Can you work these out from the model? Positions are in its coordinate system, mm. A direction names the side the tool comes from. Round coordinates to 2 decimals unless told otherwise and drop trailing zeros. Order: outer loops, then holes, each group sorted by start corner. A loop starts at its lowest first (then second) coordinate and runs counter-clockwise, first axis right, second up.
Q1. If we section it at C-C (z = 46.5): Please give me the cut outline in (x, y).
Q2. If we section it at A-A (y = 0): Please give me the cut outline in (x, z) (3 decimals), plus the area to 3 significant figures.
Q3. If we section it at B-B (x = 0): Please give me the cut outline in (y, z) (3 decimals).
Q4. Will these pins go through, and if not, where does the flat tip stop? P1, Ø16.5, axis at y = -16.5, z = 48.5, coming from the +X side; P2, Ø11.5, axis at x = -45.5, y = -11.5, coming from the +Z side; P3, Ø21.5, axis at x = 22, y = -9.5, coming from the +Z side.
Q5. We'd pull the mould along Y, two halves only. Please class faces 1 (the face through (25, 24.855, 58)), 2 (the face through (15.002, -3, 51)): pulls with the +Y half, pulls with the -Y half, needs draft (parallel to the pull), parting line crosses it, or undercut.
Q6. If we section it at D-D (z = 4): Please give me the cut outline in (x, y) (3 decimals), plus the area to 3 significant figures.
Q7. For faces 3 (the face through (-47.564, -1, 13)), 4 (the face through (58, 13.025, 13)), 5 (the face through (45, -1, 25.4)), 6 (the face through (-35.702, -2, 40)), 7 (the face through (-17.032, -40, 58)), which set-ups out of +Z, -Z, +X, -X, +Y, -Y let a thin tool reach every point of the face, with its end or its side?
Q8. If I drill on line 1 (Y direction, x = 0, z = 17) (3 decimals); line 2 (X direction, y = -41, z = 56.5); line 3 (X direction, y = 16.5, z = 49.5), over which ranges is the centre line in solid material (lowest first)?
from build123d import *

# Parameters (mm, degrees)
F0_W      = 144.9018344283
F0_H      = 100.0124998391
F1_DEPTH  = 25.4
F2_W      = 23.9564813673
F2_H      = 30.4689249024
F3_DEPTH  = 25.4
F4_W      = 27.2127054632
F4_H      = 32.7947968617
F5_DEPTH  = 25.4
F6_W      = 70.706512779
F6_H      = 100.0124998391
F7_DEPTH  = 17.78
F9_W      = 19.5373268798
F9_H      = 99.2384850979
F8_W      = 19.0721508116
F8_H      = 100.0124998391
F10_DEPTH = 10.16
F12_W     = 19.5373268798
F12_H     = 22.7496176958
F11_W     = 19.0721508116
F11_H     = 23.2910439372
F15_DEPTH = 10.16
F13_W     = 18.3743890375
F13_H     = 23.6915722489
F14_W     = 19.367502071
F14_H     = 23.0261366814
F16_DEPTH = 10.16
F19_D     = 21.59


with BuildPart() as f1:
    # F0 (on Top) → F1 (new body)
    with BuildSketch(Plane.XY):
        with Locations((-2.325873822, -1.6281101853)):
            Rectangle(F0_W, F0_H)
    extrude(amount=F1_DEPTH)

    # F2 (on face) → F3 (cut)
    with BuildSketch(Plane.XY.offset(25.4)):
        with Locations((58.1468027085, -2.2095781751)):
            Rectangle(F2_W, F2_H)
    extrude(amount=-F3_DEPTH, mode=Mode.SUBTRACT)

    # F4 (on face) → F5 (cut)
    with BuildSketch(Plane.XY.offset(25.4)):
        with Locations((-61.1704383045, -1.0466421954)):
            Rectangle(F4_W, F4_H)
    extrude(amount=-F5_DEPTH, mode=Mode.SUBTRACT)

    # F6 (on face) → F7 (join)
    with BuildSketch(Plane.XY.offset(25.4)):
        with Locations((-0.3488790244, -1.6281101853)):
            Rectangle(F6_W, F6_H)
    extrude(amount=F7_DEPTH)

    # F9 (on face) + F8 (on face) → F10 (join)
    with BuildSketch(Plane.XY.offset(43.18)):
        with Locations((24.7705369256, -2.0151175559)):
            Rectangle(F9_W, F9_H)
    with BuildSketch(Plane.XY.offset(43.18)):
        with Locations((-26.1660600081, -1.6281101853)):
            Rectangle(F8_W, F8_H)
    extrude(amount=F10_DEPTH)

    # F12 (on face) + F11 (on face) → F15 (join)
    with BuildSketch(Plane.XY.offset(53.34)):
        with Locations((24.7705369256, 36.2293161452)):
            Rectangle(F12_W, F12_H)
    with BuildSketch(Plane.XY.offset(53.34)):
        with Locations((-26.1660600081, 36.7326177657)):
            Rectangle(F11_W, F11_H)
    extrude(amount=F15_DEPTH)

    # F13 (on face) + F14 (on face) → F16 (join)
    with BuildSketch(Plane.XY.offset(53.34)):
        with Locations((-26.2195924297, -39.7885739803)):
            Rectangle(F13_W, F13_H)
    with BuildSketch(Plane.XY.offset(53.34)):
        with Locations((24.6856245212, -39.9210313335)):
            Rectangle(F14_W, F14_H)
    extrude(amount=F16_DEPTH)

    # F19 (through all)
    with Locations(Plane.XY.offset(43.18)):
        with Locations((0, 0)):
            Hole(F19_D / 2)


solid = f1.part
Solution:
1. outline: (-35.7, -51.63) - (-16.63, -51.63) - (-16.63, 48.38) - (-35.7, 48.38) - close; (15, -51.63) - (34.54, -51.63) - (34.54, 47.6) - (15, 47.6) - close
2. outline: (-47.564, 0) - (-10.795, 0) - (-10.795, 43.18) - (-16.63, 43.18) - (-16.63, 53.34) - (-35.702, 53.34) - (-35.702, 25.4) - (-47.564, 25.4) - close; (10.795, 0) - (46.169, 0) - (46.169, 25.4) - (35.004, 25.4) - (35.004, 43.18) - (34.539, 43.18) - (34.539, 53.34) - (15.002, 53.34) - (15.002, 43.18) - (10.795, 43.18) - close
2. area: 3,100 mm2
3. outline: (-51.634, 0) - (-10.795, 0) - (-10.795, 43.18) - (-51.634, 43.18) - close; (10.795, 0) - (48.378, 0) - (48.378, 43.18) - (10.795, 43.18) - close
4. P1: stops at x = 35
4. P2: stops at z = 25.4
4. P3: stops at z = 53.34
5. face 1: undercut
5. face 2: needs draft
6. outline: (-74.777, -51.634) - (70.125, -51.634) - (70.125, -17.444) - (46.169, -17.444) - (46.169, 13.025) - (70.125, 13.025) - (70.125, 48.378) - (-74.777, 48.378) - (-74.777, 15.351) - (-47.564, 15.351) - (-47.564, -17.444) - (-74.777, -17.444) - close; hole circle Ø21.59 at (0, 0)
6. area: 12,500 mm2
7. face 3: +Z, -Z, -X
7. face 4: +Z, -Z, +X
7. face 5: +Z, +X, +Y, -Y
7. face 6: +Z, -X, +Y, -Y
7. face 7: +Z, -Y
8. line 1: y = -51.634 to -10.795, 10.795 to 48.378
8. line 2: x = -35.41 to -17.03, 15 to 34.37
8. line 3: x = -35.7 to -16.63, 15 to 34.54
